The model under review builds one solid part; all positions refer to its coordinate system, in mm. A direction names the side the tool comes from. Coordinates: 2 decimals unless noted, no trailing zeros. Write each loop counter-clockwise with the first axis right and the second up, starting at its lowest first coordinate (ties: lowest second). Pieces come first, ordered by that corner, then holes.
```python
from build123d import *

# Parameters (mm, degrees)
BOSS_EXTRUDE1_DEPTH = 3.175
CUT_EXTRUDE1_DEPTH  = 3.175
FILLET1_R           = 6.35
SKETCH3_W           = 63.5
SKETCH3_H           = 3.175
BOSS_EXTRUDE2_DEPTH = 4.7625


with BuildPart() as part:
    # Sketch1 → Boss-Extrude1 (new body)
    with BuildSketch(Plane(origin=(0, 0, 0), x_dir=(1, 0, 0), z_dir=(0, 1, 0))):
        Polygon((-119.32539, 0), (-246.32539, 0), (-25.4, 303.52288513), (0, 303.52288513), align=None)
    extrude(amount=BOSS_EXTRUDE1_DEPTH)

    # Sketch2 → Cut-Extrude1 (cut)
    with BuildSketch(Plane(origin=(0, 3.175, 0), x_dir=(1, 0, 0), z_dir=(0, 1, 0))):
        Polygon((-136.632122874, 25.4), (-66.411730064, 204.016606412), (-196.421509772, 25.4), align=None)
    extrude(amount=-CUT_EXTRUDE1_DEPTH, mode=Mode.SUBTRACT)

    # Fillet1
    fillet1_edges = [part.edges().sort_by_distance(p)[0] for p in [
        (-136.632122874, 1.5875, -25.4),
        (-196.421509772, 1.5875, -25.4),
        (-66.411730064, 1.5875, -204.016606412),
    ]]
    fillet(fillet1_edges, radius=FILLET1_R)

    # Sketch3 → Boss-Extrude2 (add)
    with BuildSketch(Plane.XY):
        with Locations((-182.82539, 1.5875)):
            Rectangle(SKETCH3_W, SKETCH3_H)
    extrude(amount=BOSS_EXTRUDE2_DEPTH)


solid = part.part
```
Item 1: Mouldability with a two-part tool opening along Z and no side actions: class faces 3 (the face through (-137.409, 1.565, -149.637)), 4 (the face through (-123, 0, -139)), 5 (the face through (-189.56, 1.57, -28.78)) as pulls with the +Z half, pulls with the -Z half, needs draft (parallel to the pull), parting line crosses it, or undercut.
Solved:
face 3: pulls with the -Z half
face 4: needs draft
face 5: undercut
Item 2: Take a section at A-A, the plane y = 2.45. Write out the cut boundary in (x, z).
Solved:
outline: (-246.33, 0) - (-25.4, -303.52) - (0, -303.52) - (-119.33, 0) - (-151.08, 0) - (-151.08, 4.76) - (-214.58, 4.76) - (-214.58, 0) - close; hole (-189.08, -35.49) - (-95.61, -163.91) arc R6.35 ccw to (-84.56, -157.85) - (-135.05, -29.43) arc R6.35 ccw to (-140.96, -25.4) - (-183.95, -25.4) arc R6.35 ccw to start
Item 3: Machinability: for faces 1 (the face through (-141.689, 1.61, -100.596)), 2 (the face through (-58.827, 1.565, -153.886)), which of the approach directions +Z, -Z, +X, -X, +Y, -Y give a long, thin tool a straight path to every point of the face, cutting with its end or side? Answer none if there is none.
Solved:
face 1: +Y, -Y
face 2: +Z, +X, +Y, -Y
Item 4: For pin 1 (1.6 mm diameter, centred on x = -136.5, y = 2, fed in from +Z); pin 2 (1 mm diameter, centred on y = 1.5, z = 1.5, fed in from +X); pin 3 (1.6 mm diameter, centred on x = -161, y = 1.5, fed in from -Z), all flat-tipped, find the tip position at first contact; note any pin that passes through.
Solved:
pin 1: stops at z = 0
pin 2: stops at x = -151.08
pin 3: stops at z = -118.33
Item 5: To check wall thickness, follow line 1 along X through (y, z) = (1.45, -109); line 2 along Z through (x, y) = (-160.5, 2.5); line 3 along Z through (x, y) = (-152, 2.85). State the ranges of each line that lie inside material, in increasing order.
Solved:
line 1: x = -166.99 to -135.57, -103.77 to -76.47
line 2: z = -117.91 to -74.75, -25.4 to 4.76
line 3: z = -129.59 to -86.43, -25.4 to 4.76
Item 6: Take a section at C-C, the plane z = -48. Write out the cut boundary in (x, y) (3 decimals), plus the area to 3 significant figures.
Solved:
outline: (-211.388, 0) - (-179.972, 0) - (-179.972, 3.175) - (-211.388, 3.175) - close; (-127.747, 0) - (-100.455, 0) - (-100.455, 3.175) - (-127.747, 3.175) - close
area: 186 mm2
Item 7: Take a section at B-B, the plane x = -159.5. Write out the cut boundary in (y, z) (1 decimal).
Solved:
outline: (0, -119.3) - (3.2, -119.3) - (3.2, -76.1) - (0, -76.1) - close; (0, -25.4) - (3.2, -25.4) - (3.2, 4.8) - (0, 4.8) - close
Item 8: Take a section at D-D, the plane z = -194. Write out the cut boundary in (x, y) (1 decimal).
Solved:
outline: (-105.1, 0) - (-43.1, 0) - (-43.1, 3.2) - (-105.1, 3.2) - close
